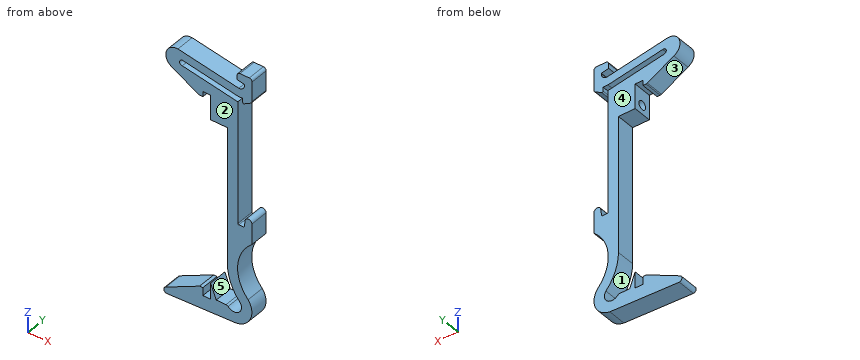
Autodesk Inventor part; units mm, degrees
ref_plane "YZ Plane" through (0, 0, 0) normal (1, 0, 0) x (0, 1, 0)
ref_plane "XZ Plane" through (0, 0, 0) normal (0, 1, 0) x (-1, 0, 0)
ref_plane "XY Plane" through (0, 0, 0) normal (0, 0, 1) x (1, 0, 0)
sketch "Sketch1" plane through (0, 0, 0) normal (0, 1, 0) x (-1, 0, 0)
  arc A0 (-159.7794, 702.6597) -> (-160.5669, 701.8721) centre (-159.7794, 701.8721) ccw
  line L0 (-155.7462, 702.6597) -> (-155.7462, 704.2667)
  line L1 (-155.7462, 704.2667) -> (-153.5139, 704.2667)
  line L2 (-153.5139, 704.2667) -> (-153.5139, 702.7873)
  line L3 (-153.5139, 702.7873) -> (-152.617, 702.7873)
  arc A1 (-164.1836, 648.4268) -> (-160.5669, 657.8731) centre (-174.7114, 657.8731) ccw
  line L4 (-160.5669, 657.8731) -> (-160.5669, 701.8721)
  arc A2 (-160.1794, 645.8656) -> (-160.7583, 645.6139) centre (-160.1783, 645.0714) ccw
  arc A3 (-164.1836, 648.4268) -> (-160.7583, 645.6139) centre (-162.4137, 647.0901) ccw
  line L5 (-155.7462, 648) -> (-155.7462, 645.3343)
  line L6 (-155.7462, 645.3343) -> (-153.4959, 645.3343)
  line L7 (-153.4959, 645.3343) -> (-153.4959, 647.6194)
  arc A4 (-143.0505, 641.0266) -> (-142.8499, 642.7649) centre (-143.1474, 641.9185) ccw
  line L8 (-163.0481, 641.9081) -> (-143.0505, 641.0266)
  arc A5 (-166.527, 650.2868) -> (-163.0481, 641.9081) centre (-162.4027, 647.0877) ccw
  arc A6 (-166.527, 650.2868) -> (-167.6435, 666.7468) centre (-174.834, 657.9912) ccw
  arc A7 (-163.8545, 670.6656) -> (-163.5889, 670.9316) centre (-163.8582, 670.9349) ccw
  line L9 (-163.5889, 706.0242) -> (-163.5889, 706.0613)
  line L10 (-163.5889, 706.0613) -> (-147.5669, 708.9022)
  arc A8 (-147.5669, 708.9022) -> (-147.8202, 710.4852) centre (-147.6004, 709.7086) ccw
  line L11 (-147.8202, 710.4852) -> (-163.5831, 707.6952)
  line L12 (-163.5831, 707.6952) -> (-164.9831, 707.6944)
  line L13 (-164.9831, 707.6944) -> (-164.9826, 706.5463)
  arc A9 (-165.396, 706.3271) -> (-164.9826, 706.5463) centre (-165.2521, 706.5552) ccw
  line L14 (-165.396, 706.3271) -> (-167.2486, 707.3943)
  arc A10 (-167.6628, 708.0983) -> (-167.2486, 707.3943) centre (-166.8615, 708.0959) ccw
  line L15 (-167.6628, 708.0983) -> (-167.6658, 713.6939)
  arc A11 (-166.8627, 714.4991) -> (-167.6658, 713.6939) centre (-166.8611, 713.6943) ccw
  line L16 (-166.8627, 714.4991) -> (-164.1837, 714.5007)
  arc A12 (-163.3795, 713.6976) -> (-164.1837, 714.5007) centre (-164.1848, 713.6954) ccw
  line L17 (-163.3795, 713.6976) -> (-163.3787, 712.3581)
  line L18 (-163.3787, 712.3581) -> (-165.5216, 711.9789)
  line L19 (-165.5216, 711.9789) -> (-165.5215, 711.7106)
  arc A13 (-165.5215, 711.7106) -> (-163.8456, 710.1095) centre (-163.9177, 711.7116) ccw
  line L20 (-163.8456, 710.1095) -> (-146.318, 713.1891)
  arc A14 (-144.6103, 707.1134) -> (-146.318, 713.1891) centre (-146.0422, 709.9888) ccw
  arc A15 (-152.617, 702.7873) -> (-152.2474, 702.8795) centre (-152.6236, 703.6003) ccw
  line L21 (-155.7462, 702.6597) -> (-155.7462, 700.1597)
  line L22 (-155.7462, 700.1597) -> (-156.9462, 700.1597)
  line L23 (-156.9462, 700.1597) -> (-157.7628, 702.6597)
  line L24 (-157.7628, 702.6597) -> (-159.7794, 702.6597)
  line L25 (-155.7462, 648) -> (-155.7462, 650)
  line L26 (-155.7462, 650) -> (-157.3545, 645.8656)
  line L27 (-157.3545, 645.8656) -> (-160.1794, 645.8656)
  line L28 (-144.6103, 707.1134) -> (-152.2474, 702.8795)
  line L29 (-152.5619, 647.6194) -> (-153.4959, 647.6194)
  line L30 (-163.8545, 670.6656) -> (-165.2545, 670.6656)
  arc A16 (-165.4084, 670.8401) -> (-165.2545, 670.6656) centre (-165.2322, 670.8403) ccw
  line L31 (-163.5889, 670.9316) -> (-163.5889, 706.0613)
  line L32 (-165.4084, 670.8401) -> (-165.7258, 673.0171)
  line L33 (-167.6435, 666.7468) -> (-167.6435, 672.6833)
  line L34 (-142.8499, 642.7649) -> (-152.5619, 647.6194)
  arc A17 (-165.7258, 673.0171) -> (-167.6435, 672.6833) centre (-166.6444, 672.619) ccw
  point P0 (-160.5669, 683.588)
  dimension "d2" = 43.999
  dimension "d6" = 2.5
  dimension "d7" = 1.2
  dimension "d8" = 2
  dimension "d18" = 1.4
  dimension "d20" = 2.2
  dimension "d21" = 1.4
  dimension "d22" = 4.0546
extrude "Extrusion1" add sketch "Sketch1" along normal blind 5.3
sketch "Sketch2" plane through (0, 0, 0) normal (0, -1, 0) x (1, 0, 0)
  line L0 (156.9462, 700.1597) -> (155.7462, 700.1597)
  line L1 (155.7462, 700.1597) -> (155.7462, 697.1597)
  line L2 (155.7462, 697.1597) -> (160.5669, 697.1597)
  line L3 (160.5669, 657.8731) -> (160.5669, 701.8721)
  line L4 (160.5669, 697.1597) -> (160.5783, 702.6397)
  line L5 (160.5783, 702.6397) -> (155.7462, 704.198)
  line L6 (155.7462, 704.198) -> (155.7462, 700.1597)
  point P0 (0, 0)
  dimension "d9" = 3
extrude "Extrusion2" add sketch "Sketch2" against normal blind 5.3
sketch "Sketch3" plane through (155.7462, 0, 704.2667) normal (-1, 0, 0) x (0, 0, 1)
  circle A0 centre (-4.5576, 2.65) radius 1.25
  line L0 (-7.107, 5.3) -> (0, 5.3)
  line L1 (0, 0) -> (-7.107, 0)
  point P0 (-704.2667, 0)
  dimension "d12" = 2.5
  dimension "d14" = 2.65
  dimension "d15" = 2.65
extrude "Extrusion3" cut sketch "Sketch3" against normal blind 5
properties part number "raspDinClipmmv4"
Can you work these out from the model? Positions are in its coordinate system, mm. Face numbers are marked on the shaded views. A direction names the side the tool comes from. Round coordinates to 2 decimals unless told otherwise and drop trailing zeros. Order: outer loops, then holes, each group sorted by start corner. A loop starts at its lowest first (then second) coordinate and runs counter-clockwise, first axis right, second up. Notation, with made-up numbers: (76.5, -33) -> (119.5, -33) arc R21 ccw to (119.5, 2) -> close; hole circle Ø2 at (36.25, -24). An arc over 180 degrees is marked (long way). Return JSON: item names as keys, results as strings. Group by question number.
1. If we section it at A-A, the plane z = 678.5: Write out the boundary of the cut face in (x, y).
2. We'd pull the mould along Z, two halves only. Please class the marked faces 1 and 2: released by +Z, released by -Z, zero draft, split by the parting line, or undercut.
3. I need wall thicknesses on line 1 (Z direction, x = 149, y = 4.95); line 2 (Z direction, x = 148.5, y = 0.2); line 3 (X direction, y = 4.25, z = 670.5). Which ranges of each line are inside material? Lowest first, please. Write a range as [from, to].
4. Will these pins go through, and if not, where does the flat tip stop? pin 1 (1.3 mm diameter, centred on y = 3, z = 707, fed in from -X); pin 2 (1.1 mm diameter, centred on x = 154.5, y = 3.5, fed in from -Z); pin 3 (1.8 mm diameter, centred on x = 154.5, y = 2.5, fed in from +Z).
5. Which directions (+Z, -Z, +X, -X, +Y, -Y) give clear straight access to the entire face, cutting with the end or side of a thin tool? Please do the marked faces 3, 4 and 5.
6. If we section it at B-B, the plane z = 659.5: Write out the boundary of the cut face in (x, y).
Output values:
{
 "1": {"outline": "(160.57, 0) -> (163.59, 0) -> (163.59, 5.3) -> (160.57, 5.3) -> close"},
 "2": {"face 1": "undercut", "face 2": "zero draft"},
 "3": {"line 1": "[641.29, 645.84], [704.68, 708.65], [710.28, 712.72]", "line 2": "[641.27, 645.59], [704.96, 708.74], [710.36, 712.81]", "line 3": "[160.57, 167.64]"},
 "4": {"pin 1": "x = 143.84", "pin 2": "z = 641.51", "pin 3": "z = 711.91"},
 "5": {"face 3": "-X, +Y, -Y", "face 4": "+Z, -Z, +X, -X, +Y", "face 5": "+Y, -Y"},
 "6": {"outline": "(160.57, 0) -> (163.61, 0) -> (163.61, 5.3) -> (160.57, 5.3) -> close"}
}
